Check sheet for the modelled part. Datum: model origin and axes. Units: mm. Round coordinates to 2 decimals unless told otherwise and drop trailing zeros. Write each loop counter-clockwise with the first axis right and the second up, starting at its lowest first coordinate (ties: lowest second). Pieces come first, ordered by that corner, then holes. Notation, with made-up numbers: (11.5, 42) -> (41.5, 42) arc R25 cw to (41.5, 74) -> close; hole circle Ø7 at (42.25, 81). An arc over 180 degrees is marked (long way). One line per item, written item: value.
from build123d import *

# Parameters (mm, degrees)
SKETCH1_R           = 1.5875
BOSS_EXTRUDE1_DEPTH = 3.175


with BuildPart() as part:
    # Sketch1 → Boss-Extrude1 (new body)
    with BuildSketch(Plane.XY):
        with BuildLine():
            Line((-0.3175, 4.1275), (11.1125, 4.1275))
            Line((11.1125, 4.1275), (4.7625, -249.8725))
            Line((4.7625, -249.8725), (-7.9375, -249.8725))
            Line((-7.9375, -249.8725), (-7.9375, -3.4925))
            ThreePointArc((-7.9375, -3.4925), (-5.705653673, 1.895653673), (-0.3175, 4.1275))
        make_face()
        Circle(SKETCH1_R, mode=Mode.SUBTRACT)
        with Locations((0, -7.62)):
            Circle(SKETCH1_R, mode=Mode.SUBTRACT)
    extrude(amount=BOSS_EXTRUDE1_DEPTH)


solid = part.part
Item 1: Depth check by flat-ended pin: pin 1 (4 mm diameter, centred on x = 0, y = -7.62, fed in from +Z) (3 decimals). Enter the tip coordinate at first touch or a pass-through.
Result set:
pin 1: z = 3.175
Item 2: Sectioned sample at A-A (z = 0.6). Enter the section's corners in (x, y) (1 decimal).
Result set:
outline: (-7.9, -249.9) -> (4.8, -249.9) -> (11.1, 4.1) -> (-0.3, 4.1) arc R7.6 ccw to (-7.9, -3.5) -> close; hole circle Ø3.2 at (0, -7.6); hole circle Ø3.2 at (0, 0)
Item 3: Release check for a two-part mould opening along Z. For faces 1 (the flat face through (0, -121, 0)), 2 (the flat face through (0, -121, 3.175)), 3 (the cylindrical face through (-5.8, 1.8, 1.6)) record: pulls with the +Z half, pulls with the -Z half, needs draft (parallel to the pull), parting line crosses it, or undercut.
Result set:
face 1: pulls with the -Z half
face 2: pulls with the +Z half
face 3: needs draft
Item 4: Sectioned sample at C-C (y = -39). Enter the section's corners in (x, z) (1 decimal).
Result set:
outline: (-7.9, 0) -> (10, 0) -> (10, 3.2) -> (-7.9, 3.2) -> close
Item 5: Material ranges on line 1 along Y through (x, z) = (0, 0.75); line 2 along Y through (x, z) = (-4, 0.75); line 3 along X through (y, z) = (-15, 0.2), recorded low to high.
Result set:
line 1: -249.87 to -9.21, -6.03 to -1.59, 1.59 to 4.13
line 2: -249.87 to 3.18
line 3: -7.94 to 10.63
Item 6: Sectioned sample at B-B (y = -214.5). Enter the section's corners in (x, z) (1 decimal), then the cut area to 3 significant figures.
Result set:
outline: (-7.9, 0) -> (5.6, 0) -> (5.6, 3.2) -> (-7.9, 3.2) -> close
area: 43.1 mm^2
